Model file for the job. Use its own axes, mm. Face numbers are marked on the shaded views. A direction names the side the tool comes from. Give positions to 0.01 mm unless a question says otherwise; leave off trailing zeros. Loops run counter-clockwise (first coordinate to the right, second up) from the corner with the lowest first, then second, coordinate; pieces in that order, holes last. Notation, with made-up numbers: M 82.5,22 L 107.5,22 A17 ccw 107.5,33 Z; hole C -38.75,84 d3. An arc over 180 degrees is marked long. Answer in a Markdown table with one row per item.
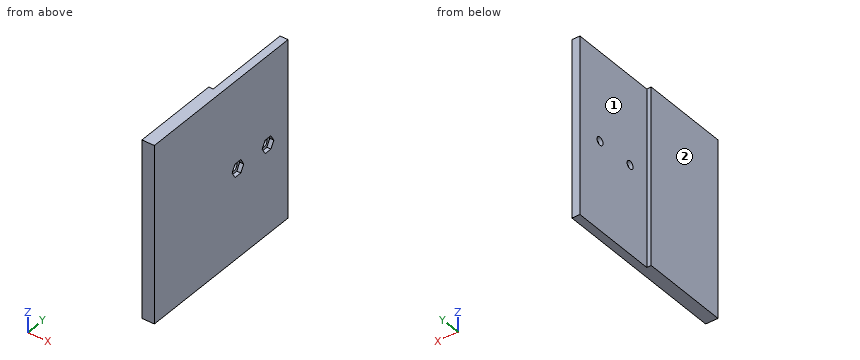
Autodesk Inventor part; units mm, degrees
ref_plane "YZ Plane" through (0, 0, 0) normal (1, 0, 0) x (0, 1, 0)
ref_plane "XZ Plane" through (0, 0, 0) normal (0, 1, 0) x (-1, 0, 0)
ref_plane "XY Plane" through (0, 0, 0) normal (0, 0, 1) x (1, 0, 0)
sketch "Sketch1" plane through (0, 0, 0) normal (1, 0, 0) x (0, 1, 0)
  line L0 (50, 50) -> (-50, 50)
  line L1 (-50, 50) -> (-50, -50)
  line L2 (-50, -50) -> (50, -50)
  line L3 (50, -50) -> (50, 50)
  point P0 (0, 0)
  point P1 (50, 0)
  point P2 (0, -50)
  dimension "d0" = 100
  dimension "d1" = 100
extrude "Extrusion1" add sketch "Sketch1" along normal blind 4.5
sketch "Sketch2" plane through (0, 0, 0) normal (-1, 0, 0) x (0, 0, 1)
  line L0 (50, -50) -> (-50, -50)
  line L1 (50, 50) -> (50, -50)
  line L2 (-50, -50) -> (50, -50)
  line L3 (50, -50) -> (50, 0)
  line L4 (50, 0) -> (-50, 0)
  line L5 (-50, 0) -> (-50, -50)
  point P0 (0, 0)
extrude "Extrusion2" add sketch "Sketch2" along normal blind 2.5
sketch "Sketch3" plane through (4.5, 0, 0) normal (1, 0, 0) x (0, 0, -1)
  line L0 (-50, -50) -> (50, -50)
  line L1 (50, -50) -> (50, 50)
  line L2 (50, 50) -> (-50, 50)
  line L3 (-50, 50) -> (-50, -50)
  point P0 (0, 0)
  point P1 (0, 35)
  point P2 (0, 12.5)
  point P3 (0, 50)
  dimension "d6" = 37.5
  dimension "d7" = 15
hole "Hole1" at (4.5, 35, 0) at (4.5, 12.5, 0) direction (-1, 0, 0) diameter 4.5 end through all
sketch "Sketch4" plane through (4.5, 0, 0) normal (1, 0, 0) x (0, 0, -1)
  circle A0 centre (0, 35) radius 2.25
  circle A1 centre (0, 12.5) radius 2.25
  line L0 (-50, -50) -> (50, -50)
  line L1 (50, -50) -> (50, 50)
  line L2 (50, 50) -> (-50, 50)
  line L3 (-50, 50) -> (-50, -50)
  line L4 (3.75, 10.3349) -> (0, 8.1699)
  line L5 (0, 8.1699) -> (-3.75, 10.3349)
  line L6 (-3.75, 10.3349) -> (-3.75, 14.6651)
  line L7 (-3.75, 14.6651) -> (0, 16.8301)
  line L8 (0, 16.8301) -> (3.75, 14.6651)
  line L9 (3.75, 14.6651) -> (3.75, 10.3349)
  line L10 (3.75, 32.8349) -> (0, 30.6699)
  line L11 (0, 30.6699) -> (-3.75, 32.8349)
  line L12 (-3.75, 32.8349) -> (-3.75, 37.1651)
  line L13 (-3.75, 37.1651) -> (0, 39.3301)
  line L14 (0, 39.3301) -> (3.75, 37.1651)
  line L15 (3.75, 37.1651) -> (3.75, 32.8349)
  point P0 (0, 0)
  dimension "d15" = 7.5
  dimension "d16" = 7.5
extrude "Extrusion3" cut sketch "Sketch4" against normal blind 2.25 contours L4 L5 L6 L7 L8 L9 | L10 L11 L12 L13 L14 L15
equation "\"d16\" = d15"
properties part number "wallMountBottom"
Q1. Drop flat-ended pins along their axis: pin 1 (2 mm diameter, centred on y = 11, z = -0.5, fed in from +X); pin 2 (15 mm diameter, centred on y = 21, z = 22, fed in from -X); pin 3 (2.5 mm diameter, centred on y = 12.5, z = 0, fed in from -X); pin 4 (2 mm diameter, centred on x = -1.5, z = -12, fed in from +Y). Give the stop position or say it passes through.
Reported:
| item | result |
|---|---|
| pin 1 | x = 2.25 |
| pin 2 | x = 0 |
| pin 3 | through |
| pin 4 | y = 0 |
Q2. Saw through at A-A (y = 35). Give the cut face in (x, z).
Reported:
| item | result |
|---|---|
| outline | M 0,-50 L 4.5,-50 L 4.5,-3.75 L 2.25,-3.75 L 2.25,-2.25 L 0,-2.25 Z; M 0,2.25 L 2.25,2.25 L 2.25,3.75 L 4.5,3.75 L 4.5,50 L 0,50 Z |
Q3. 3-axis set-ups, long thin cutter, end or side, ignore diameter. For the marked faces 1 and 2: which of +Z, -Z, +X, -X, +Y, -Y reach the whole face in a straight line?
Reported:
| item | result |
|---|---|
| face 1 | +Z, -Z, -X, +Y |
| face 2 | +Z, -Z, -X, +Y, -Y |
Q4. Probe probe 1 along Y at (x, z) = (0.75, 0); probe 2 along Z at (x, y) = (0.65, 35); probe 3 along Z at (x, y) = (3.25, 13.5). List the from-to ranges inside material, lowest first.
Reported:
| item | result |
|---|---|
| probe 1 | -50 to 10.25, 14.75 to 32.75, 37.25 to 50 |
| probe 2 | -50 to -2.25, 2.25 to 50 |
| probe 3 | -50 to -3.75, 3.75 to 50 |
Q5. Saw through at B-B (z = 33). Give the cut face in (x, y).
Reported:
| item | result |
|---|---|
| outline | M -2.5,-50 L 4.5,-50 L 4.5,50 L 0,50 L 0,0 L -2.5,0 Z |
